```python
from build123d import *

# Parameters (mm, degrees)
SKETCH2_R           = 14.2875
SKETCH2_R_2         = 3.175
BOSS_EXTRUDE1_DEPTH = 3.175


with BuildPart() as part:
    # Sketch2 → Boss-Extrude1 (new body)
    with BuildSketch(Plane(origin=(0, 0, 0), x_dir=(0, 0, -1), z_dir=(1, 0, 0))):
        with BuildLine():
            Line((-30.668144985, 154.267504682), (-42.344097145, 110.692257994))
            Line((-42.344097145, 110.692257994), (-42.344097145, 95.25))
            Line((-42.344097145, 95.25), (28.575, 95.25))
            ThreePointArc((28.575, 95.25), (30.82006403, 96.17993597), (31.75, 98.425))
            Line((31.75, 98.425), (31.75, 110.608066701))
            Line((31.75, 110.608066701), (31.75, 146.05))
            ThreePointArc((31.75, 146.05), (4.144206603, 177.528374349), (-30.668144985, 154.267504682))
        make_face()
        with Locations((0, 146.05)):
            Circle(SKETCH2_R, mode=Mode.SUBTRACT)
        with Locations((-25.4, 111.125)):
            Circle(SKETCH2_R_2, mode=Mode.SUBTRACT)
        with Locations((12.7, 111.125)):
            Circle(SKETCH2_R_2, mode=Mode.SUBTRACT)
    extrude(amount=BOSS_EXTRUDE1_DEPTH)


solid = part.part
```
Geometry check sheet. Reference: the model listing, model coordinates, mm. Round coordinates to 2 decimals unless told otherwise and drop trailing zeros. Loops run counter-clockwise (first coordinate to the right, second up) from the corner with the lowest first, then second, coordinate; pieces in that order, holes last. Notation, with made-up numbers: (72.25, 55.25) - (79.25, 55.25) arc R11 ccw to (79.25, 76.25) - close; hole circle Ø9 at (86.25, 14). An arc over 180 degrees is marked (long way). Use a Markdown table: item, result.
Q1. Cross-section at D-D on z = -12.7. Record the cut outline in (x, y) (3 decimals).
Solutions:
| item | result |
|---|---|
| outline | (0, 95.25) - (3.175, 95.25) - (3.175, 107.95) - (0, 107.95) - close; (0, 114.3) - (3.175, 114.3) - (3.175, 139.505) - (0, 139.505) - close; (0, 152.595) - (3.175, 152.595) - (3.175, 175.149) - (0, 175.149) - close |
Q2. Draft check along Y on faces 1 (the flat face through (1.565, 132.785, 36.424)), 2 (the cylindrical face through (1.565, 160.216, 1.86)), 3 (the flat face through (2, 122, -31.75)). Enter one of: released by +Y, released by -Y, zero draft, split by the parting line, or undercut.
Solutions:
| item | result |
|---|---|
| face 1 | released by +Y |
| face 2 | undercut |
| face 3 | zero draft |
Q3. Cross-section at C-C on y = 141.5. Record the cut outline in (x, z) (3 decimals).
Solutions:
| item | result |
|---|---|
| outline | (0, -31.75) - (3.175, -31.75) - (3.175, -13.544) - (0, -13.544) - close; (0, 13.544) - (3.175, 13.544) - (3.175, 34.089) - (0, 34.089) - close |
Q4. Go/stop test with a flat-tipped pin: P1, Ø5.5, axis at y = 111.125, z = 25.4, coming from the -X side. Record where the tip stops, or that it passes through.
Solutions:
| item | result |
|---|---|
| P1 | passes through |
Q5. Cross-section at B-B on x = 2.15. State how many separate pieces and enclosed holes the cut face has, plus the area to 3 significant figures.
Solutions:
| item | result |
|---|---|
| separate pieces | 1 |
| enclosed holes | 3 |
| area | 4,480 mm2 |
Q6. Material ranges on line 1 (Y direction, x = 2, z = -12); line 2 (Y direction, x = 2, z = 0); line 3 (Y direction, x = 0.9, z = -12.7), recorded low to high.
Solutions:
| item | result |
|---|---|
| line 1 | y = 95.25 to 108.03, 114.22 to 138.3, 153.8 to 175.44 |
| line 2 | y = 95.25 to 131.76, 160.34 to 177.8 |
| line 3 | y = 95.25 to 107.95, 114.3 to 139.5, 152.6 to 175.15 |
